from build123d import *

# Parameters (mm, degrees)
F1_DEPTH = 3.5
F3_DEPTH = 2.4
F4_D     = 3.3


with BuildPart() as f1:
    # F0 (on Top) → F1 (new body)
    with BuildSketch(Plane.XY):
        Polygon((0, 5), (-1.164685703, 4.3466662183), (-2.5, 4.3301270189), (-3.1819805153, 3.1819805153), (-4.3301270189, 2.5), (-4.3466662183, 1.164685703), (-5, 0), (-4.3466662183, -1.164685703), (-4.3301270189, -2.5), (-3.1819805153, -3.1819805153), (-2.5, -4.3301270189), (-1.164685703, -4.3466662183), (0, -5), (1.164685703, -4.3466662183), (2.5, -4.3301270189), (3.1819805153, -3.1819805153), (4.3301270189, -2.5), (4.3466662183, -1.164685703), (5, 0), (4.3466662183, 1.164685703), (4.3301270189, 2.5), (3.1819805153, 3.1819805153), (2.5, 4.3301270189), (1.164685703, 4.3466662183), align=None)
    extrude(amount=F1_DEPTH)

    # F2 (on face) → F3 (cut)
    with BuildSketch(Plane.XY.offset(3.5)):
        Polygon((-1.6454482672, -2.85), (1.6454482672, -2.85), (3.2908965344, 0), (1.6454482672, 2.85), (-1.6454482672, 2.85), (-3.2908965344, 0), align=None)
    extrude(amount=-F3_DEPTH, mode=Mode.SUBTRACT)

    # F4 (through all)
    with Locations(Plane(origin=(0, 0, 0), x_dir=(1, 0, 0), z_dir=(0, 0, -1))):
        with Locations((0, 0)):
            Hole(F4_D / 2)


solid = f1.part
The model under review builds one solid part; all positions refer to its coordinate system, in mm. A direction names the side the tool comes from. Round coordinates to 2 decimals unless told otherwise and drop trailing zeros. Order: outer loops, then holes, each group sorted by start corner. A loop starts at its lowest first (then second) coordinate and runs counter-clockwise, first axis right, second up. Notation, with made-up numbers: (24, 81) - (69, 81) arc R25 ccw to (69, 99) - close; hole circle Ø3 at (-7.75, -22). An arc over 180 degrees is marked (long way). Use one line per item in the form item = value.
Q1. Mouldability with a two-part tool opening along X and no side actions: class faces 3 (the flat face through (-3.76, -2.84, 1.73)), 4 (the flat face through (2.84, -3.76, 1.73)), 5 (the flat face through (1.4, 1.3, 1.1)) as pulls with the +X half, pulls with the -X half, needs draft (parallel to the pull), parting line crosses it, or undercut.
Response values:
face_3 = pulls with the -X half
face_4 = pulls with the +X half
face_5 = undercut
Q2. Add section D-D on y = 2. Give the boundary of the cut face in (x, z).
Response values:
outline = (-4.34, 0) - (4.34, 0) - (4.34, 3.5) - (2.14, 3.5) - (2.14, 1.1) - (-2.14, 1.1) - (-2.14, 3.5) - (-4.34, 3.5) - close
Q3. Clearance check with flat-ended pins moving along their axes: P1, Ø1, axis at x = -1, z = 0.5, coming from the +Y side; P2, Ø5.5, axis at x = 0, y = 0, coming from the +Z side; P3, Ø1.5, axis at y = -3.5, z = 2.5, coming from the -X side. State where each tip first meets the part, or that it passes through.
Response values:
P1 = 4.72
P2 = 1.1
P3 = -3.91
Q4. Add section A-A on y = -0.75. Give the boundary of the cut face in (x, z), then the cut area to 3 significant figures.
Response values:
outline = (-4.58, 0) - (-1.47, 0) - (-1.47, 1.1) - (-2.86, 1.1) - (-2.86, 3.5) - (-4.58, 3.5) - close; (1.47, 0) - (4.58, 0) - (4.58, 3.5) - (2.86, 3.5) - (2.86, 1.1) - (1.47, 1.1) - close
area = 15.1 mm^2
Q5. Tool access review of faces 1 (the flat face through (-0.57, 4.68, 1.73)), 2 (the flat face through (-2.48, -1.405, 2.317)): name each direction out of +Z, -Z, +X, -X, +Y, -Y from which nothing blocks a thin tool from reaching the whole face with its end or side.
Response values:
face_1 = +Z, -Z, -X, +Y
face_2 = +Z
Q6. Add section B-B on x = 1. Give the boundary of the cut face in (y, z).
Response values:
outline = (-4.44, 0) - (-1.31, 0) - (-1.31, 1.1) - (-2.85, 1.1) - (-2.85, 3.5) - (-4.44, 3.5) - close; (1.31, 0) - (4.44, 0) - (4.44, 3.5) - (2.85, 3.5) - (2.85, 1.1) - (1.31, 1.1) - close
Q7. To check wall thickness, follow line 1 (X direction, y = -1.5, z = 2.5); line 2 (X direction, y = 2, z = 2.6); line 3 (Y direction, x = 3, z = 3.35). State the ranges of each line that lie inside material, in increasing order.
Response values:
line_1 = -4.34 to -2.42, 2.42 to 4.34
line_2 = -4.34 to -2.14, 2.14 to 4.34
line_3 = -3.49 to -0.5, 0.5 to 3.49
